```python
from build123d import *

# Parameters (mm, degrees)
BASE_EXTRUDE_DEPTH  = 76.2
BOSS_EXTRUDE2_DEPTH = 59.427356
SKETCH4_W           = 70
SKETCH4_H           = 70
BOSS_EXTRUDE3_DEPTH = 451.60000000000053
FILLET1_START       = -36.936387435
FILLET1_DEPTH       = 431.8
FILLET1_2_OUTLINE_W = 451.6
FILLET1_2_OUTLINE_H = 70
FILLET1_2_DEPTH     = 70
FILLET1_START_2     = 324.863612565
FILLET1_3_OUTLINE_W = 451.6
FILLET1_3_OUTLINE_H = 70
FILLET1_3_DEPTH     = 70
FILLET2_R           = 19.999999999999996
FILLET4_R           = 9.999999999999996
FILLET7_R           = 9.999999999999996
FILLET11_R          = 40


with BuildPart() as part:
    # Sketch1 → Base-Extrude (new body)
    with BuildSketch(Plane.XY):
        Polygon((-36.93638743455497, 59.4273560209424), (394.863612565445, 59.4273560209424), (394.86361256544507, -440.5726439790576), (-36.93638743455492, -440.5726439790576), align=None)
    extrude(amount=-BASE_EXTRUDE_DEPTH)

    # Sketch3 → Boss-Extrude2 (add)
    with BuildSketch(Plane(origin=(0, 0, 0), x_dir=(1, 0, 0), z_dir=(0, 1, 0))):
        Polygon((-36.93638743455497, 76.2), (394.1216881668196, 76.2), (394.12168816681964, -342.9), (-36.93638743455493, -342.9), align=None)
    extrude(amount=BOSS_EXTRUDE2_DEPTH)

    # Sketch4 → Boss-Extrude3 (add)
    with BuildSketch(Plane(origin=(0, 59.4273560209424, 0), x_dir=(-1, 0, 0), z_dir=(0, 1, 0))):
        Polygon((36.93638743455493, 342.9), (-33.06361256544507, 342.9), (-33.06361256544506, 272.9), (36.93638743455494, 272.9), align=None)
        with Locations((-359.12168816681964, 307.9)):
            Rectangle(SKETCH4_W, SKETCH4_H)
    extrude(amount=BOSS_EXTRUDE3_DEPTH)

    # Fillet1: read off the stored shape, not the designer's step
    # Fillet1 outline → Fillet1 (cut)
    with BuildSketch(Plane.YZ.offset(FILLET1_START)):
        with BuildLine():
            Line((-440.572643979, 0), (-440.572643979, -60))
            ThreePointArc((-440.572643979, -60), (-422.99905085, -17.573593129), (-380.572643979, 0))
            Line((-380.572643979, 0), (-440.572643979, 0))
        make_face()
    extrude(amount=FILLET1_DEPTH, mode=Mode.SUBTRACT)

    # Fillet1 2 outline → Fillet1 2 (add)
    with BuildSketch(Plane.YZ.offset(FILLET1_START)):
        with Locations((285.227356021, -41.2)):
            Rectangle(FILLET1_2_OUTLINE_W, FILLET1_2_OUTLINE_H)
    extrude(amount=FILLET1_2_DEPTH)

    # Fillet1 3 outline → Fillet1 3 (add)
    with BuildSketch(Plane.YZ.offset(FILLET1_START_2)):
        with Locations((285.227356021, -41.2)):
            Rectangle(FILLET1_3_OUTLINE_W, FILLET1_3_OUTLINE_H)
    extrude(amount=FILLET1_3_DEPTH)

    # Fillet2
    fillet2_edges = [part.edges().sort_by_distance(p)[0] for p in [
        (178.59265036613232, 0, 0),
    ]]
    fillet(fillet2_edges, radius=FILLET2_R)

    # Fillet4
    fillet4_edges = [part.edges().sort_by_distance(p)[0] for p in [
        (394.12168816681964, 0, 181.45),
        (394.1216881668196, -5.857864376269045, 5.857864376269044),
    ]]
    fillet(fillet4_edges, radius=FILLET4_R)

    # Fillet7
    fillet7_edges = [part.edges().sort_by_distance(p)[0] for p in [
        (-36.93638743455492, -440.5726439790576, -68.1),
        (-36.936387435, -422.99905085, -17.573593129000002),
        (-36.936387434554945, -200.2863219895, 0),
        (-36.936387434554945, 0, 181.45),
        (-36.936387434554945, -5.857864376269045, 5.857864376269044),
    ]]
    fillet(fillet7_edges, radius=FILLET7_R)

    # Fillet11
    # the kernel refuses this fillet: 40 mm, written as the material it takes off along each edge
    with BuildSketch(Plane(origin=(484.12168816681964, 0, 342.9), x_dir=(0, 0, -1), z_dir=(-1, 0, 0))) as fillet11_piece_1:
        with BuildLine():
            CenterArc((FILLET11_R, -FILLET11_R), FILLET11_R, 90, 90)
            Line((0, -FILLET11_R), (0, 0))
            Line((0, 0), (FILLET11_R, 0))
        make_face()
    extrude(amount=611.0580756013748, mode=Mode.SUBTRACT)


solid = part.part
```
Here's how the part is built. I have some questions about the finished solid (model axes, mm). A direction names the side the tool comes from. Coordinates: 2 decimals unless noted, no trailing zeros. Loops run counter-clockwise (first coordinate to the right, second up) from the corner with the lowest first, then second, coordinate; pieces in that order, holes last. Notation, with made-up numbers: (31.5, -28) - (49.5, -28) arc R22 ccw to (49.5, -5) - close; hole circle Ø9 at (9, -36.5). An arc over 180 degrees is marked (long way). Return JSON: item names as keys, results as strings. Group by question number.
Item 1: If we section it at B-B on x = 126.5: Write out the boundary of the cut face in (y, z).
Item 2: I need wall thicknesses on line 1 (Z direction, x = -4.5, y = 451.5); line 2 (X direction, y = 416, z = 306); line 3 (Z direction, x = 37.5, y = -104.5). Which ranges of each line are inside material? Lowest first, please. Write a range as from..to.
Item 3: Will these pins go through, and if not, where does the flat tip stop? P1, Ø1, axis at x = 291, y = -311, coming from the +Z side; P2, Ø1.5, axis at x = 229, z = 108.5, coming from the +Y side; P3, Ø10, axis at x = 181.5, z = 62, coming from the -Y side.
Item 4: We'd pull the mould along X, two halves only. Please class faces 1 (the face through (360, 511.027, 308)), 2 (the face through (394.864, 29, -38)), 3 (the face through (324.122, 282, 307)): +X half, -X half, draft (parallel to the pull), parting line (faces both ways), or undercut.
Item 5: On a 3-axis mill with a long thin cutter (end or side, diameter ignored), from which of +Z, -Z, +X, -X, +Y, -Y can I reach the whole of each face in a straight line? I mean faces 4 (the face through (-1, 282, 272.9)), 5 (the face through (33.064, 282, -41)), 6 (the face through (181, 0, 159)). Say none if no direction works.
Item 6: If we section it at A-A on y = 275.5: Write out the boundary of the cut face in (x, z), and give its area (3 significant figures).
Item 7: If we section it at D-D on y = -302: Write out the boundary of the cut face in (x, z), and give its area (3 significant figures).
Item 8: If we section it at C-C on z = 226: Write out the boundary of the cut face in (x, y).
Calculated:
{
 "1": {"outline": "(-440.57, -76.2) - (59.43, -76.2) - (59.43, 342.9) - (40, 342.9) arc R40 ccw to (0, 302.9) - (0, 20) arc R20 cw to (-20, 0) - (-380.57, 0) arc R60 ccw to (-440.57, -60) - close"},
 "2": {"line 1": "z = -76.2..-6.2, 272.9..342.9", "line 2": "x = -36.94..33.06, 324.12..394.12", "line 3": "z = -76.2..0"},
 "3": {"P1": "stops at z = 0", "P2": "stops at y = 59.43", "P3": "stops at y = 0"},
 "4": {"face 1": "draft", "face 2": "+X half", "face 3": "undercut"},
 "5": {"face 4": "+X, -X, +Y", "face 5": "+Z, -Z, +Y", "face 6": "+Z, +X, -X, -Y"},
 "6": {"outline": "(-36.94, -76.2) - (33.06, -76.2) - (33.06, -6.2) - (-36.94, -6.2) - close; (-36.94, 272.9) - (33.06, 272.9) - (33.06, 342.9) - (-36.94, 342.9) - close; (324.12, 272.9) - (394.12, 272.9) - (394.12, 342.9) - (324.12, 342.9) - close; (324.86, -76.2) - (394.86, -76.2) - (394.86, -6.2) - (324.86, -6.2) - close", "area": "19,600 mm^2"},
 "7": {"outline": "(-36.94, -76.2) - (394.86, -76.2) - (394.86, 0) - (-26.94, 0) arc R10 ccw to (-36.94, -10) - close", "area": "32,900 mm^2"},
 "8": {"outline": "(-36.94, 10) arc R10 ccw to (-26.94, 0) - (384.12, 0) arc R10 ccw to (394.12, 10) - (394.12, 59.43) - (-36.94, 59.43) - close"}
}
